The model under review builds one solid part; all positions refer to its coordinate system, in mm. Face numbers are marked on the shaded views. A direction names the side the tool comes from. Coordinates: 2 decimals unless noted, no trailing zeros. Write each loop counter-clockwise with the first axis right and the second up, starting at its lowest first coordinate (ties: lowest second). Pieces come first, ordered by that corner, then holes.
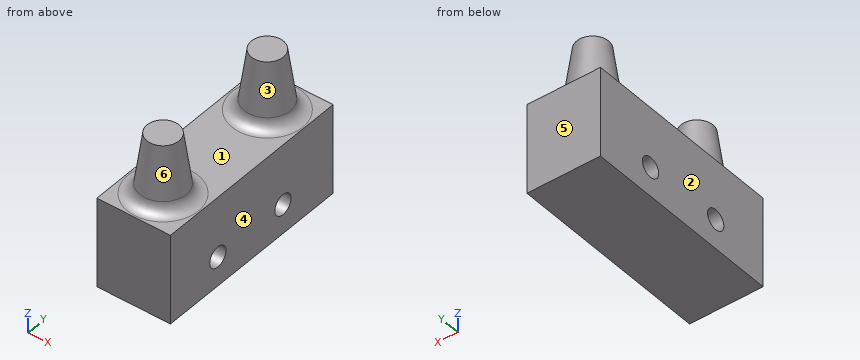
```python
from build123d import *

# Parameters (mm, degrees)
BOSS_EXTRUDE1_DEPTH           = 22
SKETCH3_R                     = 6
BOSS_EXTRUDE3_DEPTH           = 15
BOSS_EXTRUDE3_DRAFT           = 8
BOSS_EXTRUDE3_PROFILE_2_DEPTH = 15
BOSS_EXTRUDE3_PROFILE_2_DRAFT = 8
FILLET2_R                     = 3
SKETCH4_R                     = 2.500012638
CUT_EXTRUDE1_DEPTH            = 50
SKETCH5_R                     = 2.500012638
CUT_EXTRUDE2_DEPTH            = 50


with BuildPart() as part:
    # Sketch2 → Boss-Extrude1 (new body)
    with BuildSketch(Plane.XY):
        Polygon((697.707943159, -649.017765949), (697.707943159, -690.080887605), (715.655949844, -690.080887605), (715.655949844, -640.080811229), (697.707943159, -640.080811229), align=None)
    extrude(amount=-BOSS_EXTRUDE1_DEPTH)


with BuildPart() as boss_extrude3_tool:
    # Sketch3 → Boss-Extrude3 (with draft: the straight prism first)
    with BuildSketch(Plane.XY):
        with Locations((706.707943159, -649.017765949)):
            Circle(SKETCH3_R)
    extrude(amount=BOSS_EXTRUDE3_DEPTH)
    # Boss-Extrude3: the draft: its side faces are tilted about the plane it starts from
    boss_extrude3_sides = [boss_extrude3_tool.faces().sort_by_distance(p)[0] for p in [
        (700.707943159, -649.017765949, 7.5),
    ]]
    draft(boss_extrude3_sides, Plane.XY, BOSS_EXTRUDE3_DRAFT)


with BuildPart() as part_1:
    add(part.part)

    # Boss-Extrude3: add boss_extrude3_tool
    add(boss_extrude3_tool.part)


with BuildPart() as boss_extrude3_profile_2_tool:
    # Sketch3 → Boss-Extrude3 profile 2 (with draft: the straight prism first)
    with BuildSketch(Plane.XY):
        with Locations((706.707943159, -681.085054274)):
            Circle(SKETCH3_R)
    extrude(amount=BOSS_EXTRUDE3_PROFILE_2_DEPTH)
    # Boss-Extrude3 profile 2: the draft: its side faces are tilted about the plane it starts from
    boss_extrude3_profile_2_sides = [boss_extrude3_profile_2_tool.faces().sort_by_distance(p)[0] for p in [
        (700.707943159, -681.085054274, 7.5),
    ]]
    draft(boss_extrude3_profile_2_sides, Plane.XY, BOSS_EXTRUDE3_PROFILE_2_DRAFT)


with BuildPart() as part_2:
    add(part_1.part)

    # Boss-Extrude3 profile 2: add boss_extrude3_profile_2_tool
    add(boss_extrude3_profile_2_tool.part)

    # Fillet2
    fillet2_edges = [part_2.edges().sort_by_distance(p)[0] for p in [
        (700.707943159, -649.017765949, 0),
        (700.707943159, -681.085054274, 0),
    ]]
    fillet(fillet2_edges, radius=FILLET2_R)

    # Sketch4 → Cut-Extrude1 (cut)
    with BuildSketch(Plane(origin=(715.655949844, 0, 0), x_dir=(0, 0, -1), z_dir=(1, 0, 0))):
        with Locations((14.80020958, -655.486173041)):
            Circle(SKETCH4_R)
    extrude(amount=-CUT_EXTRUDE1_DEPTH, mode=Mode.SUBTRACT)

    # Sketch5 → Cut-Extrude2 (cut)
    with BuildSketch(Plane(origin=(715.655949844, 0, 0), x_dir=(0, 0, -1), z_dir=(1, 0, 0))):
        with Locations((14.80020958, -675.510263036)):
            Circle(SKETCH5_R)
    extrude(amount=-CUT_EXTRUDE2_DEPTH, mode=Mode.SUBTRACT)


solid = part_2.part
```
Item 1: Take a section at A-A, the plane z = -16.5. Write out the cut boundary in (x, y).
Solved:
outline: (697.71, -690.08) - (715.66, -690.08) - (715.66, -677.34) - (697.71, -677.34) - close; (697.71, -673.68) - (715.66, -673.68) - (715.66, -657.32) - (697.71, -657.32) - close; (697.71, -653.65) - (715.66, -653.65) - (715.66, -640.08) - (697.71, -640.08) - close
Item 2: Take a section at C-C, the plane x = 705. Count the separate pieces of the cut face and the enclosed holes in it, plus the area to 3 significant figures.
Solved:
separate pieces: 1
enclosed holes: 2
area: 1,340 mm2
Item 3: Mouldability with a two-part tool opening along Y and no side actions: class the marked faces 3, 4, 5 and 6 as pulls with the +Y half, pulls with the -Y half, needs draft (parallel to the pull), parting line crosses it, or undercut.
Solved:
face 3: undercut
face 4: needs draft
face 5: pulls with the +Y half
face 6: undercut
Item 4: To check wall thickness, follow line 1 along Y through (x, z) = (708, -15.5); line 2 along Z through (x, y) = (701.25, -661.5); line 3 along Z through (x, y) = (704, -673.5). State the ranges of each line that lie inside material, in increasing order.
Solved:
line 1: y = -690.08 to -677.91, -673.11 to -657.89, -653.09 to -640.08
line 2: z = -22 to 0
line 3: z = -22 to -16.29, -13.31 to 0.05
Item 5: Take a section at D-D, the plane z = 6.5. Write out the cut boundary in (x, y), plus the area to 3 significant figures.
Solved:
outline: circle Ø10.17 at (706.71, -681.09); circle Ø10.17 at (706.71, -649.02)
area: 163 mm2
Item 6: Machinability: for the marked faces 1 and 2, which of the approach directions +Z, -Z, +X, -X, +Y, -Y give a long, thin tool a straight path to every point of the face, cutting with its end or side? Answer none if there is none.
Solved:
face 1: +Z
face 2: +Z, -Z, -X, +Y, -Y
Item 7: For pin 1 (6 mm diameter, centred on x = 710, y = -678, fed in from +Z); pin 2 (3 mm diameter, centred on x = 706, z = 2.5, fed in from -Y), all flat-tipped, find the tip position at first contact; note any pin that passes through.
Solved:
pin 1: stops at z = 15
pin 2: stops at y = -687.43
Item 8: Take a section at B-B, the plane y = -664.5. Write out the cut boundary in (x, z).
Solved:
outline: (697.71, -22) - (715.66, -22) - (715.66, 0) - (697.71, 0) - close
